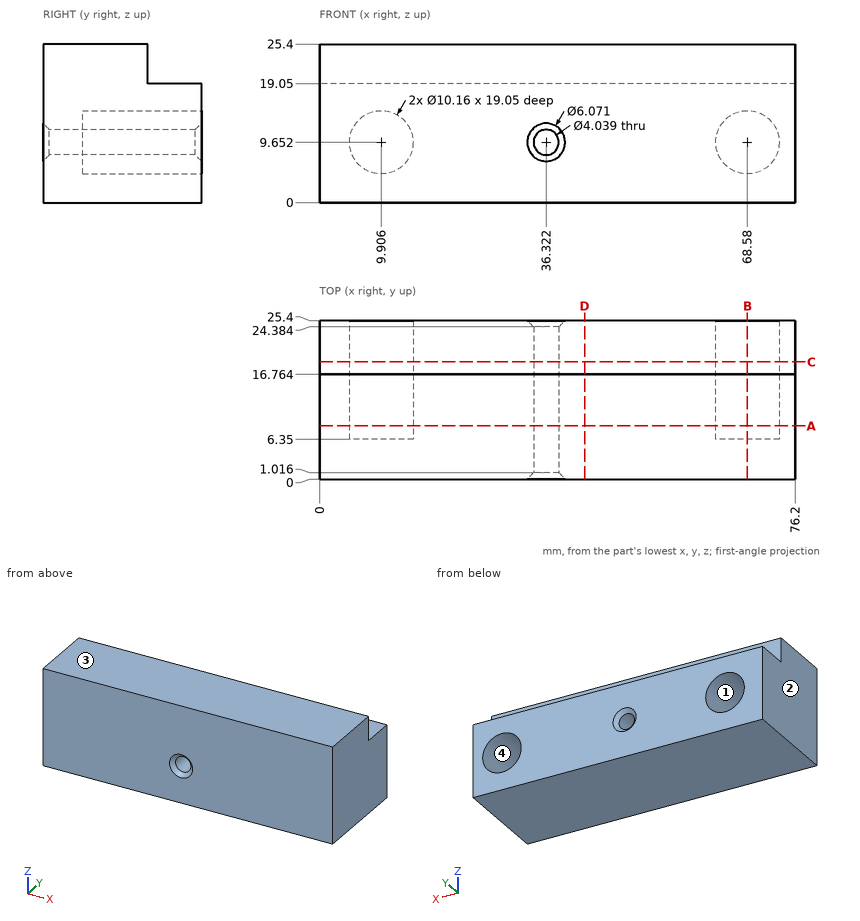
Geometry: see drawing. Coordinates: mm, zero at the bounding-box minimum. Coordinates: 2 decimals unless noted, no trailing zeros. Loops run counter-clockwise (first coordinate to the right, second up) from the corner with the lowest first, then second, coordinate; pieces in that order, holes last. Notation, with made-up numbers: M -14,20.5 L 9,20.5 A12 cw 9,28.5 Z; hole C -6.5,4 d3. An arc over 180 degrees is marked long. Answer in a Markdown table with one row per item.
Q1. Section D-D on x = 42.5. Return the cut outline in (y, z), plus the area to 3 significant figures.
Answers below:
| item | result |
|---|---|
| outline | M 0,0 L 25.4,0 L 25.4,19.05 L 16.76,19.05 L 16.76,25.4 L 0,25.4 Z |
| area | 590 mm^2 |
Q2. First-contact query: pin 1 (5 mm diameter, centred on x = 67, z = 8, fed in from +Y); pin 2 (1.9 mm diameter, centred on x = 44.5, z = 21.5, fed in from +Y). Flat tips, straight axial feed; report the tip coordinate or a pass-through.
Answers below:
| item | result |
|---|---|
| pin 1 | stops at y = 6.35 |
| pin 2 | stops at y = 16.76 |
Q3. Ray query, probe 1 along Z at (x, y) = (68.58, 11.25); probe 2 along X at (y, z) = (20.25, 5.25) (1 decimal); probe 3 along Y at (x, z) = (62, 19.5). Return the intervals inside material, ascending. Write a range as from..to.
Answers below:
| item | result |
|---|---|
| probe 1 | z = 0..4.57, 14.73..25.4 |
| probe 2 | x = 0..7.4, 12.4..66, 71.1..76.2 |
| probe 3 | y = 0..16.76 |
Q4. Section B-B on x = 68.58. Return the cut outline in (y, z).
Answers below:
| item | result |
|---|---|
| outline | M 0,0 L 25.4,0 L 25.4,4.57 L 6.35,4.57 L 6.35,14.73 L 25.4,14.73 L 25.4,19.05 L 16.76,19.05 L 16.76,25.4 L 0,25.4 Z |
Q5. Section A-A on y = 8.5. Return the cut outline in (x, z), plus the area to 3 significant figures.
Answers below:
| item | result |
|---|---|
| outline | M 0,0 L 76.2,0 L 76.2,25.4 L 0,25.4 Z; hole C 9.91,9.65 d10.16; hole C 36.32,9.65 d4.04; hole C 68.58,9.65 d10.16 |
| area | 1,760 mm^2 |
Q6. Draft query along Z for the marked faces 1, 2, 3 and 4. Return one class per face: pulls with the +Z half, pulls with the -Z half, needs draft (parallel to the pull), parting line crosses it, or undercut.
Answers below:
| item | result |
|---|---|
| face 1 | undercut |
| face 2 | needs draft |
| face 3 | pulls with the +Z half |
| face 4 | undercut |
Q7. Section C-C on y = 18.75. Return the cut outline in (x, z), plus the area to 3 significant figures.
Answers below:
| item | result |
|---|---|
| outline | M 0,0 L 76.2,0 L 76.2,19.05 L 0,19.05 Z; hole C 9.91,9.65 d10.16; hole C 36.32,9.65 d4.04; hole C 68.58,9.65 d10.16 |
| area | 1,280 mm^2 |
